from build123d import *

# Parameters (mm, degrees)
BOSS_EXTRUDE1_DEPTH     = 600
M36_TAPPED_HOLE1_D      = 32
CUT_EXTRUDE1_DEPTH      = 928.36184955
CUT_EXTRUDE1_DEPTH_BACK = 100
SKETCH6_R               = 10
CUT_EXTRUDE2_START      = -100
SKETCH7_R               = 10
CUT_EXTRUDE2_DEPTH      = 100


with BuildPart() as part:
    # Sketch1 → Boss-Extrude1 (new body)
    with BuildSketch(Plane.XY):
        Polygon((110, 0), (390, 0), (390, 100), (500, 100), (500, 400), (390, 400), (390, 500), (110, 500), (110, 400), (0, 400), (0, 100), (110, 100), align=None)
    extrude(amount=BOSS_EXTRUDE1_DEPTH)

    # M36 Tapped Hole1 (through all)
    with Locations(Plane(origin=(0, 100, 0), x_dir=(-1, 0, 0), z_dir=(0, -1, 0))):
        with Locations((-50, -50), (-50, -550), (-450, -50), (-450, -550)):
            Hole(M36_TAPPED_HOLE1_D / 2)

    # Sketch6 → Cut-Extrude1 (cut, two sides: drawn at the far end of the back side and taken through both)
    with BuildSketch(Plane(origin=(500, 0, 0), x_dir=(0, 0, -1), z_dir=(1, 0, 0)).offset(-CUT_EXTRUDE1_DEPTH_BACK)):
        with Locations(Location((-300, 150, 0), (0, 0, 180))):
            Circle(SKETCH6_R)
        with Locations(Location((-300, 350, 0), (0, 0, 180))):
            Circle(SKETCH6_R)
    extrude(amount=CUT_EXTRUDE1_DEPTH + CUT_EXTRUDE1_DEPTH_BACK, mode=Mode.SUBTRACT)

    # Sketch7 → Cut-Extrude2 (cut)
    with BuildSketch(Plane.ZY.offset(CUT_EXTRUDE2_START)):
        with Locations((300, 150)):
            Circle(SKETCH7_R)
        with Locations((300, 350)):
            Circle(SKETCH7_R)
    extrude(amount=CUT_EXTRUDE2_DEPTH, mode=Mode.SUBTRACT)


solid = part.part
Geometry: final body of the model. Coordinates: model frame, mm. A direction names the side the tool comes from. Round coordinates to 2 decimals unless told otherwise and drop trailing zeros. Loops run counter-clockwise (first coordinate to the right, second up) from the corner with the lowest first, then second, coordinate; pieces in that order, holes last. Notation, with made-up numbers: M 84,14.5 L 101,14.5 A21 cw 101,32.5 Z; hole C 57.5,5 d2. An arc over 180 degrees is marked long. Put each result on its own line as item: value. Start each with the question number.
(1) Draft query along Z for faces 1 (the face through (449.3, 340.085, 298.698)), 2 (the face through (247, 254, 0)), 3 (the face through (500, 248, 296)), 4 (the face through (247, 254, 600)). Return one class per face: +Z half, -Z half, draft (parallel to the pull), parting line (faces both ways), or undercut.
(2) Contact query for flat-ended pins moving along their axis: pin 1 Ø16 at (y, z) = (148.5, 300) entering from -X; pin 2 Ø19 at (x, z) = (450, 550) entering from +Y. Output: stop coordinate, or through.
(3) Section query A-A (x = 450). Return loops of the section in (y, z).
(4) Set-up query: faces 5 (the face through (110, 451, 296)), 6 (the face through (390, 449, 296)), 7 (the face through (400, 350, 300)), 8 (the face through (444, 100, 296)), 9 (the face through (51, 144, 292)). Return all of +Z, -Z, +X, -X, +Y, -Y with unobstructed straight access to the full face (end or side cutting, diameter ignored); none if empty.
(5) Material intervals for line 1 along X through (y, z) = (279, 550); line 2 along Z through (x, y) = (450, 207); line 3 along Y through (x, z) = (74, 300), sorted ascending. Write a range as [from, to].
(6) Section query C-C (z = 550). Return loops of the section in (x, y), then the cut area to 3 significant figures.
(7) Section query D-D (z = 320.5). Return loops of the section in (x, y).
(8) Section query B-B (y = 150). Return loops of the section in (x, z).
Findings below:
1. face 1: undercut
1. face 2: -Z half
1. face 3: draft
1. face 4: +Z half
2. pin 1: stops at x = 100
2. pin 2: passes through
3. outline: M 100,0 L 400,0 L 400,34 L 100,34 Z; M 100,66 L 400,66 L 400,534 L 100,534 Z; M 100,566 L 400,566 L 400,600 L 100,600 Z; hole C 150,300 d20; hole C 350,300 d20
4. face 5: +Z, -Z, -X, +Y
4. face 6: +Z, -Z, +X, +Y
4. face 7: +X
4. face 8: +Z, -Z, +X, -Y
4. face 9: -X
5. line 1: x = [0, 34], [66, 434], [466, 500]
5. line 2: z = [0, 34], [66, 534], [566, 600]
5. line 3: y = [100, 140], [160, 340], [360, 400]
6. outline: M 0,100 L 34,100 L 34,400 L 0,400 Z; M 66,100 L 110,100 L 110,0 L 390,0 L 390,100 L 434,100 L 434,400 L 390,400 L 390,500 L 110,500 L 110,400 L 66,400 Z; M 466,100 L 500,100 L 500,400 L 466,400 Z
6. area: 187,000 mm2
7. outline: M 0,100 L 110,100 L 110,0 L 390,0 L 390,100 L 500,100 L 500,400 L 390,400 L 390,500 L 110,500 L 110,400 L 0,400 Z
8. outline: M 0,0 L 500,0 L 500,290 L 400,290 L 400,310 L 500,310 L 500,600 L 0,600 L 0,310 L 100,310 L 100,290 L 0,290 Z; hole C 50,50 d32; hole C 50,550 d32; hole C 450,50 d32; hole C 450,550 d32
